Work out the finished part from the listing and answer in its coordinate system (mm). Face numbers are marked on the shaded views. Coordinates: 2 decimals unless noted, no trailing zeros. Order: outer loops, then holes, each group sorted by start corner. A loop starts at its lowest first (then second) coordinate and runs counter-clockwise, first axis right, second up. Notation, with made-up numbers: M -19,58 L -7,58 A20 ccw -7,89 Z; hole C -14.75,62 d11. An arc over 180 degrees is marked long. Use a Markdown table: item, result.
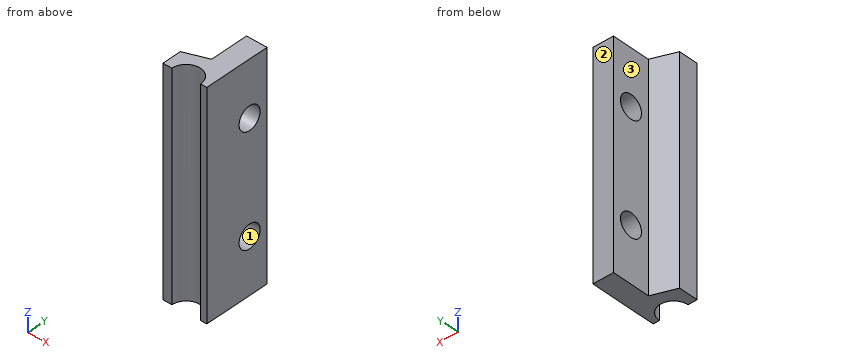
from build123d import *

# Parameters (mm, degrees)
BOSS_EXTRUDE1_DEPTH = 40
SKETCH2_R           = 2.1
CUT_EXTRUDE1_DEPTH  = 42.990351999


with BuildPart() as part:
    # Sketch1 → Boss-Extrude1 (new body)
    with BuildSketch(Plane.XY):
        with BuildLine():
            Line((-2.6, 0), (-4.25, 0))
            Line((-4.25, 0), (-4.25, 3.5))
            Line((-4.25, 3.5), (0, 5.046873496))
            Line((0, 5.046873496), (0, 12.046873496))
            Line((0, 12.046873496), (3.75, 12.046873496))
            Line((3.75, 12.046873496), (3.75, 0))
            Line((3.75, 0), (2.6, 0))
            ThreePointArc((2.6, 0), (0, 2.6), (-2.6, 0))
        make_face()
    extrude(amount=BOSS_EXTRUDE1_DEPTH)

    # Sketch2 → Cut-Extrude1 (cut, through all)
    with BuildSketch(Plane.ZY):
        with Locations((10, 8.546873496)):
            Circle(SKETCH2_R)
        with Locations((30, 8.546873496)):
            Circle(SKETCH2_R)
    extrude(amount=-CUT_EXTRUDE1_DEPTH, mode=Mode.SUBTRACT)


solid = part.part
(1) Given P1, Ø5, axis at y = 9, z = 19, coming from the -X side; P2, Ø3.5, axis at y = 8.55, z = 10, coming from the -X side, each flat-ended and moving along its own axis, determine where each tip first touches the part or whether it passes through.
Conclusion:
| item | result |
|---|---|
| P1 | x = 0 |
| P2 | through |
(2) Straight lines are drawn through the part: L1, parallel to Y at x = 2.95, z = 10; L2, parallel to Z at x = 1.5, y = 9; L3, parallel to X at y = 11, z = 15. For each, find the intervals that lie inside material, in ascending order.
Conclusion:
| item | result |
|---|---|
| L1 | 0 to 6.45, 10.65 to 12.05 |
| L2 | 0 to 7.95, 12.05 to 27.95, 32.05 to 40 |
| L3 | 0 to 3.75 |
(3) A cutting plane is placed at A-A (z = 30). Determine the outline of the cut face in (x, y).
Conclusion:
| item | result |
|---|---|
| outline | M -4.25,0 L -2.6,0 A2.6 cw 2.6,0 L 3.75,0 L 3.75,6.45 L 0,6.45 L 0,5.05 L -4.25,3.5 Z; M 0,10.65 L 3.75,10.65 L 3.75,12.05 L 0,12.05 Z |
(4) A cutting plane is placed at D-D (y = 1.25). Determine the outline of the cut face in (x, z).
Conclusion:
| item | result |
|---|---|
| outline | M -4.25,0 L -2.28,0 L -2.28,40 L -4.25,40 Z; M 2.28,0 L 3.75,0 L 3.75,40 L 2.28,40 Z |
(5) A cutting plane is placed at C-C (z = 4). Determine the outline of the cut face in (x, y), then the cut area to 3 significant figures.
Conclusion:
| item | result |
|---|---|
| outline | M -4.25,0 L -2.6,0 A2.6 cw 2.6,0 L 3.75,0 L 3.75,12.05 L 0,12.05 L 0,5.05 L -4.25,3.5 Z |
| area | 52.7 mm2 |
(6) A cutting plane is placed at B-B (y = 7). Determine the outline of the cut face in (x, z).
Conclusion:
| item | result |
|---|---|
| outline | M 0,0 L 3.75,0 L 3.75,8.58 L 0,8.58 Z; M 0,11.42 L 3.75,11.42 L 3.75,28.58 L 0,28.58 Z; M 0,31.42 L 3.75,31.42 L 3.75,40 L 0,40 Z |
(7) Determine the mould class of the marked faces 1, 2 and 3 for opening direction Y: pulls with the +Y half, pulls with the -Y half, needs draft (parallel to the pull), parting line crosses it, or undercut.
Conclusion:
| item | result |
|---|---|
| face 1 | undercut |
| face 2 | pulls with the +Y half |
| face 3 | needs draft |
